```python
from build123d import *

# Parameters (mm, degrees)
SKETCH1_W           = 196.85
SKETCH1_H           = 120
BOSS_EXTRUDE1_DEPTH = 3.175
SKETCH2_W           = 152.4
SKETCH2_H           = 2.188710325
SKETCH2_W_2         = 3.175
SKETCH2_H_2         = 3.175
CUT_EXTRUDE3_DEPTH  = 3.175
BOSS_EXTRUDE3_DEPTH = 3.175
CUT_EXTRUDE5_DEPTH  = 6.175
BOSS_EXTRUDE4_DEPTH = 3.175
SKETCH8_W           = 16.66875
SKETCH8_H           = 1
CUT_EXTRUDE6_DEPTH  = 4
SKETCH9_W           = 16.66875
SKETCH9_H           = 1
CUT_EXTRUDE7_DEPTH  = 4


with BuildPart() as part:
    # Sketch1 → Boss-Extrude1 (new body)
    with BuildSketch(Plane(origin=(0, 0, 0), x_dir=(1, 0, 0), z_dir=(0, 1, 0))):
        Rectangle(SKETCH1_W, SKETCH1_H)
    extrude(amount=BOSS_EXTRUDE1_DEPTH)

    # Sketch2 → Cut-Extrude3 (cut)
    with BuildSketch(Plane(origin=(0, 0, 0), x_dir=(1, 0, 0), z_dir=(0, 1, 0))):
        with BuildLine():
            ThreePointArc((-87.55, -42.045183145), (-86.085533906, -38.509649239), (-82.55, -37.045183145))
            Line((-82.55, -37.045183145), (-98.425, -37.045183145))
            Line((-98.425, -37.045183145), (-98.425, -57.045183145))
            Line((-98.425, -57.045183145), (-82.55, -57.045183145))
            ThreePointArc((-82.55, -57.045183145), (-86.085533906, -55.580717051), (-87.55, -52.045183145))
            Line((-87.55, -52.045183145), (-87.55, -42.045183145))
        make_face()
        Polygon((-82.55, -37.045183145), (-76.2, -37.045183145), (-76.2, -18.966736095), (-82.55, -18.966736095), (-98.425, -18.966736095), (-98.425, -37.045183145), align=None)
        with BuildLine():
            Line((-98.425, -18.966736095), (-82.55, -18.966736095))
            ThreePointArc((-82.55, -18.966736095), (-86.085533906, -17.502270001), (-87.55, -13.966736095))
            Line((-87.55, -13.966736095), (-87.55, 6.033263905))
            ThreePointArc((-87.55, 6.033263905), (-86.085533906, 9.568797811), (-82.55, 11.033263905))
            Line((-82.55, 11.033263905), (-98.425, 11.033263905))
            Line((-98.425, 11.033263905), (-98.425, -18.966736095))
        make_face()
        with BuildLine():
            Line((-76.2, 11.033263905), (-76.2, 42.808053265))
            Line((-76.2, 42.808053265), (-92.86875, 42.808053265))
            Line((-92.86875, 42.808053265), (-96.04375, 42.808053265))
            ThreePointArc((-96.04375, 42.808053265), (-97.276375702, 42.970331517), (-98.425, 43.44610728))
            Line((-98.425, 43.44610728), (-98.425, 11.033263905))
            Line((-98.425, 11.033263905), (-82.55, 11.033263905))
            Line((-82.55, 11.033263905), (-79.375, 11.033263905))
            Line((-79.375, 11.033263905), (-76.2, 11.033263905))
        make_face()
        with BuildLine():
            Line((-92.86875, 57.811289675), (-76.2, 57.811289675))
            Line((-76.2, 57.811289675), (-76.2, 60))
            Line((-76.2, 60), (-98.425, 60))
            Line((-98.425, 60), (-98.425, 57.173235661))
            ThreePointArc((-98.425, 57.173235661), (-97.276375702, 57.649011423), (-96.04375, 57.811289675))
            Line((-96.04375, 57.811289675), (-92.86875, 57.811289675))
        make_face()
        with Locations((0, 58.905644838)):
            Rectangle(SKETCH2_W, SKETCH2_H)
        with BuildLine():
            Line((76.2, 60), (76.2, 57.811289675))
            Line((76.2, 57.811289675), (92.86875, 57.811289675))
            Line((92.86875, 57.811289675), (92.86875, 54.636289675))
            Line((92.86875, 54.636289675), (96.04375, 54.636289675))
            Line((96.04375, 54.636289675), (96.04375, 57.811289675))
            ThreePointArc((96.04375, 57.811289675), (97.276375702, 57.649011423), (98.425, 57.173235661))
            Line((98.425, 57.173235661), (98.425, 60))
            Line((98.425, 60), (76.2, 60))
        make_face()
        with BuildLine():
            Line((79.375, -18.966736095), (76.2, -18.966736095))
            Line((76.2, -18.966736095), (76.2, -37.045183145))
            Line((76.2, -37.045183145), (82.55, -37.045183145))
            ThreePointArc((82.55, -37.045183145), (86.085533906, -38.509649239), (87.55, -42.045183145))
            Line((87.55, -42.045183145), (87.55, -52.045183145))
            ThreePointArc((87.55, -52.045183145), (86.085533906, -55.580717051), (82.55, -57.045183145))
            Line((82.55, -57.045183145), (82.55, -53.870183145))
            Line((82.55, -53.870183145), (79.375, -53.870183145))
            Line((79.375, -53.870183145), (79.375, -57.045183145))
            Line((79.375, -57.045183145), (76.2, -57.045183145))
            Line((76.2, -57.045183145), (76.2, -59.23389347))
            Line((76.2, -59.23389347), (76.2, -60))
            Line((76.2, -60), (98.425, -60))
            Line((98.425, -60), (98.425, 0))
            Line((98.425, 0), (98.425, 43.44610728))
            ThreePointArc((98.425, 43.44610728), (97.276375702, 42.970331517), (96.04375, 42.808053265))
            Line((96.04375, 42.808053265), (96.04375, 45.983053265))
            Line((96.04375, 45.983053265), (92.86875, 45.983053265))
            Line((92.86875, 45.983053265), (92.86875, 42.808053265))
            Line((92.86875, 42.808053265), (87.3125, 42.808053265))
            Line((87.3125, 42.808053265), (76.2, 42.808053265))
            Line((76.2, 42.808053265), (76.2, 11.033263905))
            Line((76.2, 11.033263905), (79.375, 11.033263905))
            Line((79.375, 11.033263905), (79.375, 7.858263905))
            Line((79.375, 7.858263905), (82.55, 7.858263905))
            Line((82.55, 7.858263905), (82.55, 11.033263905))
            ThreePointArc((82.55, 11.033263905), (86.085533906, 9.568797811), (87.55, 6.033263905))
            Line((87.55, 6.033263905), (87.55, -13.966736095))
            ThreePointArc((87.55, -13.966736095), (86.085533906, -17.502270001), (82.55, -18.966736095))
            Line((82.55, -18.966736095), (79.375, -18.966736095))
        make_face()
        Polygon((76.2, -59.23389347), (76.2, -57.045183145), (-76.2, -57.045183145), (-76.2, -59.23389347), (-76.2, -60), (76.2, -60), align=None)
        Polygon((-76.2, -59.23389347), (-76.2, -57.045183145), (-79.375, -57.045183145), (-82.55, -57.045183145), (-98.425, -57.045183145), (-98.425, -60), (-76.2, -60), align=None)
        with Locations((-80.9625, -55.457683145)):
            Rectangle(SKETCH2_W_2, SKETCH2_H_2)
        with Locations((-80.9625, 9.445763905)):
            Rectangle(SKETCH2_W_2, SKETCH2_H_2)
        with Locations((-94.45625, 44.395553265)):
            Rectangle(SKETCH2_W_2, SKETCH2_H_2)
        with Locations((-94.45625, 56.223789675)):
            Rectangle(SKETCH2_W_2, SKETCH2_H_2)
    extrude(amount=CUT_EXTRUDE3_DEPTH, mode=Mode.SUBTRACT)

    # Sketch5 → Boss-Extrude3 (add)
    with BuildSketch(Plane(origin=(0, 0, 0), x_dir=(1, 0, 0), z_dir=(0, 1, 0))):
        with BuildLine():
            ThreePointArc((-98.425, 57.173235661), (-100.168195986, 55.430039675), (-100.80625, 53.048789675))
            Line((-100.80625, 53.048789675), (-100.80625, 47.570553265))
            ThreePointArc((-100.80625, 47.570553265), (-100.168195986, 45.189303265), (-98.425, 43.44610728))
            Line((-98.425, 43.44610728), (-98.425, 57.173235661))
        make_face()
        with BuildLine():
            ThreePointArc((100.80625, 53.048789675), (100.168195986, 55.430039675), (98.425, 57.173235661))
            Line((98.425, 57.173235661), (98.425, 43.44610728))
            ThreePointArc((98.425, 43.44610728), (100.168195986, 45.189303265), (100.80625, 47.570553265))
            Line((100.80625, 47.570553265), (100.80625, 53.048789675))
        make_face()
    extrude(amount=BOSS_EXTRUDE3_DEPTH)

    # Sketch6 → Cut-Extrude5 (cut)
    with BuildSketch(Plane(origin=(0, 0, 0), x_dir=(1, 0, 0), z_dir=(0, 1, 0))):
        with BuildLine():
            Line((-45.8, -18.966736095), (45.8, -18.966736095))
            ThreePointArc((45.8, -18.966736095), (49.335533906, -17.502270001), (50.8, -13.966736095))
            Line((50.8, -13.966736095), (50.8, 57.811289675))
            Line((50.8, 57.811289675), (-50.8, 57.811289675))
            Line((-50.8, 57.811289675), (-50.8, -13.966736095))
            ThreePointArc((-50.8, -13.966736095), (-49.335533906, -17.502270001), (-45.8, -18.966736095))
        make_face()
        Polygon((-50.8, -57.045183145), (-40.8, -47.045183145), (40.8, -47.045183145), (50.8, -57.045183145), align=None)
    extrude(amount=CUT_EXTRUDE5_DEPTH, mode=Mode.SUBTRACT)

    # Sketch7 → Boss-Extrude4 (add)
    with BuildSketch(Plane(origin=(0, 0, 0), x_dir=(1, 0, 0), z_dir=(0, 1, 0))):
        with BuildLine():
            Line((-50.8, 57.811289675), (-50.8, 67.811289675))
            ThreePointArc((-50.8, 67.811289675), (-52.659871939, 72.301417736), (-57.15, 74.161289675))
            Line((-57.15, 74.161289675), (-69.85, 74.161289675))
            ThreePointArc((-69.85, 74.161289675), (-74.340128061, 72.301417736), (-76.2, 67.811289675))
            Line((-76.2, 67.811289675), (-76.2, 57.811289675))
            Line((-76.2, 57.811289675), (-50.8, 57.811289675))
        make_face()
        with BuildLine():
            Line((76.2, 57.811289675), (76.2, 67.811289675))
            ThreePointArc((76.2, 67.811289675), (74.340128061, 72.301417736), (69.85, 74.161289675))
            Line((69.85, 74.161289675), (57.15, 74.161289675))
            ThreePointArc((57.15, 74.161289675), (52.659871939, 72.301417736), (50.8, 67.811289675))
            Line((50.8, 67.811289675), (50.8, 57.811289675))
            Line((50.8, 57.811289675), (76.2, 57.811289675))
        make_face()
        with BuildLine():
            ThreePointArc((-50.8, -67.045183145), (-52.659871939, -71.535311205), (-57.15, -73.395183145))
            Line((-57.15, -73.395183145), (-69.85, -73.395183145))
            ThreePointArc((-69.85, -73.395183145), (-74.340128061, -71.535311205), (-76.2, -67.045183145))
            Line((-76.2, -67.045183145), (-76.2, -57.045183145))
            Line((-76.2, -57.045183145), (-50.8, -57.045183145))
            Line((-50.8, -57.045183145), (-50.8, -67.045183145))
        make_face()
        with BuildLine():
            Line((50.8, -57.045183145), (50.8, -67.045183145))
            ThreePointArc((50.8, -67.045183145), (52.659871939, -71.535311205), (57.15, -73.395183145))
            Line((57.15, -73.395183145), (69.85, -73.395183145))
            ThreePointArc((69.85, -73.395183145), (74.340128061, -71.535311205), (76.2, -67.045183145))
            Line((76.2, -67.045183145), (76.2, -57.045183145))
            Line((76.2, -57.045183145), (50.8, -57.045183145))
        make_face()
    extrude(amount=BOSS_EXTRUDE4_DEPTH)

    # Sketch8 → Cut-Extrude6 (cut)
    with BuildSketch(Plane(origin=(0, 0, 0), x_dir=(1, 0, 0), z_dir=(0, 1, 0))):
        with Locations((84.534375, 43.308053265)):
            Rectangle(SKETCH8_W, SKETCH8_H)
        with Locations((84.534375, 57.311289675)):
            Rectangle(SKETCH8_W, SKETCH8_H)
    extrude(amount=CUT_EXTRUDE6_DEPTH, mode=Mode.SUBTRACT)

    # Sketch9 → Cut-Extrude7 (cut)
    with BuildSketch(Plane(origin=(0, 0, 0), x_dir=(1, 0, 0), z_dir=(0, 1, 0))):
        with Locations((-84.534375, 57.311289675)):
            Rectangle(SKETCH9_W, SKETCH9_H)
        with Locations((-84.534375, 43.308053265)):
            Rectangle(SKETCH9_W, SKETCH9_H)
    extrude(amount=CUT_EXTRUDE7_DEPTH, mode=Mode.SUBTRACT)


solid = part.part
```
Input: part model. Units: mm. Frame: model coordinates. A direction names the side the tool comes from. Give positions to 0.01 mm unless a question says otherwise; leave off trailing zeros. Order: outer loops, then holes, each group sorted by start corner. A loop starts at its lowest first (then second) coordinate and runs counter-clockwise, first axis right, second up. Notation, with made-up numbers: (20, -20) - (71, -20) arc R24 cw to (71, 13) - close; hole circle Ø10 at (20, 30). An arc over 180 degrees is marked (long way). One line per item, written item: value.
1. Pin query (flat end, axial travel): pin 1 Ø1.6 at (y, z) = (1, -35.5) entering from -X; pin 2 Ø1 at (y, z) = (2, -56.5) entering from -X; pin 3 Ø1.6 at (x, y) = (-80.5, 2) entering from -Z. Return the tip coordinate at first contact, or that it passes through.
Determined:
pin 1: x = -76.2
pin 2: x = -99.78
pin 3: z = -56.81
2. Reachability of faces 4 (the face through (-52.611, 1.565, 71.486)), 5 (the face through (-86.124, 1.565, -9.53)), 6 (the face through (-52.61, 1.57, -72.25)) from +Z, -Z, +X, -X, +Y, -Y: full face, straight path, thin tool, end or side. Return the list, or none.
Determined:
face 4: +Z, +Y, -Y
face 5: -X, +Y, -Y
face 6: -Z, +Y, -Y
3. Draft query along X for faces 1 (the face through (86.046, 1.565, 38.471)), 2 (the face through (49.3, 1.57, 17.54)), 3 (the face through (-74.29, 1.565, 71.584)). Return one class per face: released by +X, released by -X, zero draft, split by the parting line, or undercut.
Determined:
face 1: released by +X
face 2: undercut
face 3: released by -X
4. Cut plane A-A, the plane z = -61.5. Output: boundary loops of the cut face in (x, y) (3 decimals), and give its area (3 significant figures).
Determined:
outline: (-76.2, 0) - (-50.8, 0) - (-50.8, 3.175) - (-76.2, 3.175) - close; (50.8, 0) - (76.2, 0) - (76.2, 3.175) - (50.8, 3.175) - close
area: 161 mm2
5. Cut plane B-B, the plane x = 5.5. Output: boundary loops of the cut face in (y, z) (3 decimals).
Determined:
outline: (0, 18.967) - (3.175, 18.967) - (3.175, 47.045) - (0, 47.045) - close
6. Cut plane C-C, the plane z = 39.5. Output: boundary loops of the cut face in (x, y) (3 decimals).
Determined:
outline: (-86.854, 0) - (86.854, 0) - (86.854, 3.175) - (-86.854, 3.175) - close
7. Line query: probe 1 along Z at (x, y) = (-77, 0.5); probe 2 along X at (y, z) = (1.2, -31.5); probe 3 along Z at (x, y) = (87, 0.9). Output: solid intervals per line, ascending.
Determined:
probe 1: -56.81 to -43.81, -11.03 to 18.97, 37.05 to 57.05
probe 2: -76.2 to -50.8, 50.8 to 76.2
probe 3: -56.81 to -43.81, -8.31 to 16.25, 39.77 to 54.32
